from build123d import *

# Parameters (mm, degrees)
SKETCH_1_W               = 40
SKETCH_1_H               = 40
EXTRUDE_1_DEPTH          = 20
SKETCH_2_R               = 3
EXTRUDE_2_DEPTH          = 4.5
SKETCH_4_R               = 2
SKETCH_4_W               = 8
SKETCH_4_H               = 20
EXTRUDE_4_DEPTH          = 2.7
SKETCH_5_W               = 4
SKETCH_5_H               = 7
EXTRUDE_5_DEPTH          = 7
SKETCH_6_W               = 48
SKETCH_6_H               = 20
CUT_EXTRUDE_1_DEPTH      = 27.5
CUT_EXTRUDE_3_DEPTH      = 54.481305145
CUT_EXTRUDE_3_DEPTH_BACK = 54.481305145
SKETCH_7_W               = 40
SKETCH_7_H               = 20
SKETCH_8_W               = 56
SKETCH_8_H               = 5
EXTRUDE_6_DEPTH          = 2.7
SKETCH_9_W               = 56
SKETCH_9_H               = 25
EXTRUDE_7_DEPTH          = 30
CUT_EXTRUDE_4_DEPTH      = 62.878914018
CUT_EXTRUDE_4_DEPTH_BACK = 62.878914018
SKETCH_10_W              = 40
SKETCH_10_H              = 20
CUT_EXTRUDE_5_DEPTH      = 64.232033021
CUT_EXTRUDE_5_DEPTH_BACK = 64.232033021
SKETCH_11_R              = 2
SKETCH_11_R_2            = 2.023853946
CUT_EXTRUDE_6_DEPTH      = 75.500268456
CUT_EXTRUDE_6_DEPTH_BACK = 75.500268456
SKETCH_12_W              = 27.5
SKETCH_12_H              = 18.538560396
SKETCH_13_W              = 56
SKETCH_13_H              = 25
EXTRUDE_8_DEPTH          = 4
SKETCH_14_W              = 36.7
SKETCH_14_H              = 2
EXTRUDE_9_DEPTH          = 56
SKETCH_15_W              = 36.7
SKETCH_15_H              = 2
EXTRUDE_10_DEPTH         = 8
SKETCH_16_W              = 36.7
SKETCH_16_H              = 2
EXTRUDE_11_DEPTH         = 8
CUT_EXTRUDE_7_DEPTH      = 76.918969961
CUT_EXTRUDE_7_DEPTH_BACK = 76.918969961
SKETCH_17_W              = 40.5
SKETCH_17_H              = 30
SKETCH_20_W              = 7.75
SKETCH_20_H              = 22.78217045
CUT_EXTRUDE_9_DEPTH      = 8
SKETCH_21_R              = 1.5
CUT_EXTRUDE_10_DEPTH     = 78.515740337


with BuildPart() as part:
    # Sketch 1 → Extrude 1 (new body)
    with BuildSketch(Plane(origin=(0, 0, 0), x_dir=(1, 0, 0), z_dir=(0, 1, 0))):
        with Locations((20, 20)):
            Rectangle(SKETCH_1_W, SKETCH_1_H)
    extrude(amount=EXTRUDE_1_DEPTH)

    # Sketch 2 → Extrude 2 (add)
    with BuildSketch(Plane.XY):
        with Locations(Location((10, 10, 0), (0, 0, 180))):
            Circle(SKETCH_2_R)
    extrude(amount=EXTRUDE_2_DEPTH)

    # Sketch 4 → Extrude 4 (add)
    # profile 1 of 3: a face of its own
    with BuildSketch(Plane(origin=(0, 0, -12.3), x_dir=(-1, 0, 0), z_dir=(0, 0, -1))):
        with BuildLine():
            Line((-44.5, 17), (-44.5, 20))
            Line((-44.5, 20), (-48, 20))
            Line((-48, 20), (-48, 0))
            Line((-48, 0), (-40, 0))
            Line((-40, 0), (-40, 15))
            Line((-40, 15), (-42.5, 15))
            ThreePointArc((-42.5, 15), (-45.914213562, 13.585786438), (-44.5, 17))
        make_face()
        with Locations((-44.5, 5)):
            Circle(SKETCH_4_R, mode=Mode.SUBTRACT)
    # profile 2 of 3: a face of its own
    with BuildSketch(Plane(origin=(0, 0, -12.3), x_dir=(-1, 0, 0), z_dir=(0, 0, -1))):
        with BuildLine():
            Line((-40, 15), (-40, 20))
            Line((-40, 20), (-44.5, 20))
            Line((-44.5, 20), (-44.5, 17))
            ThreePointArc((-44.5, 17), (-43.085786438, 16.414213562), (-42.5, 15))
            Line((-42.5, 15), (-40, 15))
        make_face()
    # profile 3 of 3: a face of its own
    with BuildSketch(Plane(origin=(0, 0, -12.3), x_dir=(-1, 0, 0), z_dir=(0, 0, -1))):
        with Locations((4, 10)):
            Rectangle(SKETCH_4_W, SKETCH_4_H)
        with Locations((4.5, 5)):
            Circle(SKETCH_4_R, mode=Mode.SUBTRACT)
        with Locations((4.5, 15)):
            Circle(SKETCH_4_R, mode=Mode.SUBTRACT)
    extrude(amount=-EXTRUDE_4_DEPTH)

    # Sketch 5 → Extrude 5 (add)
    with BuildSketch(Plane.ZY):
        with Locations((-35, 10)):
            Rectangle(SKETCH_5_W, SKETCH_5_H)
    extrude(amount=EXTRUDE_5_DEPTH)

    # Sketch 6 → Cut-Extrude 1 (cut)
    with BuildSketch(Plane(origin=(0, 0, -40), x_dir=(-1, 0, 0), z_dir=(0, 0, -1))):
        with Locations((-16, 10)):
            Rectangle(SKETCH_6_W, SKETCH_6_H)
    extrude(amount=-CUT_EXTRUDE_1_DEPTH, mode=Mode.SUBTRACT)

    # Sketch 7 → Cut-Extrude 3 (cut, two sides: drawn at the far end of the back side and taken through both)
    with BuildSketch(Plane.XY.offset(-CUT_EXTRUDE_3_DEPTH_BACK)):
        with Locations((20, 10)):
            Rectangle(SKETCH_7_W, SKETCH_7_H)
    extrude(amount=CUT_EXTRUDE_3_DEPTH + CUT_EXTRUDE_3_DEPTH_BACK, mode=Mode.SUBTRACT)


with BuildPart() as cut_extrude_3_piece_1:
    # of the separate pieces the step leaves, piece 1, a body of its own (cut_extrude_3_pieces)
    add(part.part.solids().sort_by_distance((0, 20, -9.6))[0])



with BuildPart() as cut_extrude_3_piece_2:
    # of the separate pieces the step leaves, piece 2, a body of its own (cut_extrude_3_pieces)
    add(part.part.solids().sort_by_distance((40, 0, -9.6))[0])


with BuildPart() as cut_extrude_3_piece_1_1:
    add(cut_extrude_3_piece_1.part)

    add(cut_extrude_3_piece_2.part)  # Extrude 6 merges Cut-Extrude 3 piece 2
    # Sketch 8 → Extrude 6 (add)
    with BuildSketch(Plane.XY.offset(-9.6)):
        with Locations((20, 22.5)):
            Rectangle(SKETCH_8_W, SKETCH_8_H)
    extrude(amount=-EXTRUDE_6_DEPTH)

    # Sketch 9 → Extrude 7 (add)
    with BuildSketch(Plane(origin=(0, 0, -12.3), x_dir=(-1, 0, 0), z_dir=(0, 0, -1))):
        with Locations((-20, 12.5)):
            Rectangle(SKETCH_9_W, SKETCH_9_H)
    extrude(amount=EXTRUDE_7_DEPTH)

    # Sketch 10 → Cut-Extrude 4 (cut, two sides: drawn at the far end of the back side and taken through both)
    with BuildSketch(Plane.XY.offset(-12.3).offset(-CUT_EXTRUDE_4_DEPTH_BACK)):
        with Locations((20, 10)):
            Rectangle(SKETCH_10_W, SKETCH_10_H)
    extrude(amount=CUT_EXTRUDE_4_DEPTH + CUT_EXTRUDE_4_DEPTH_BACK, mode=Mode.SUBTRACT)

    # Sketch 11 → Cut-Extrude 5 (cut, two sides: drawn at the far end of the back side and taken through both)
    with BuildSketch(Plane.XY.offset(-9.6).offset(-CUT_EXTRUDE_5_DEPTH_BACK)):
        with Locations(Location((-4.5, 15, 0), (0, 0, 180))):
            Circle(SKETCH_11_R)
        with Locations(Location((-4.5, 5, 0), (0, 0, 180))):
            Circle(SKETCH_11_R)
        with Locations((44.5, 15)):
            Circle(SKETCH_11_R_2)
        with Locations(Location((44.5, 5, 0), (0, 0, 180))):
            Circle(SKETCH_11_R)
    extrude(amount=CUT_EXTRUDE_5_DEPTH + CUT_EXTRUDE_5_DEPTH_BACK, mode=Mode.SUBTRACT)

    # Sketch 12 → Cut-Extrude 6 (cut, two sides: drawn at the far end of the back side and taken through both)
    with BuildSketch(Plane(origin=(48, 0, 0), x_dir=(0, 0, -1), z_dir=(1, 0, 0)).offset(-CUT_EXTRUDE_6_DEPTH_BACK)):
        with Locations((27.459022476, 9.269280198)):
            Rectangle(SKETCH_12_W, SKETCH_12_H)
    extrude(amount=CUT_EXTRUDE_6_DEPTH + CUT_EXTRUDE_6_DEPTH_BACK, mode=Mode.SUBTRACT)

    # Sketch 13 → Extrude 8 (add)
    with BuildSketch(Plane(origin=(0, 0, -42.3), x_dir=(-1, 0, 0), z_dir=(0, 0, -1))):
        with Locations((-20, 12.5)):
            Rectangle(SKETCH_13_W, SKETCH_13_H)
    extrude(amount=EXTRUDE_8_DEPTH)

    # Sketch 14 → Extrude 9 (add)
    with BuildSketch(Plane(origin=(48, 0, 0), x_dir=(0, 0, -1), z_dir=(1, 0, 0))):
        with Locations((27.95, -1)):
            Rectangle(SKETCH_14_W, SKETCH_14_H)
    extrude(amount=-EXTRUDE_9_DEPTH)

    # Sketch 15 → Extrude 10 (add)
    with BuildSketch(Plane(origin=(48, 0, 0), x_dir=(0, 0, -1), z_dir=(1, 0, 0))):
        with Locations((27.95, -1)):
            Rectangle(SKETCH_15_W, SKETCH_15_H)
    extrude(amount=EXTRUDE_10_DEPTH)

    # Sketch 16 → Extrude 11 (add)
    with BuildSketch(Plane.ZY.offset(8)):
        with Locations((-27.95, -1)):
            Rectangle(SKETCH_16_W, SKETCH_16_H)
    extrude(amount=EXTRUDE_11_DEPTH)

    # Sketch 17 → Cut-Extrude 7 (cut, two sides: drawn at the far end of the back side and taken through both)
    with BuildSketch(Plane.XZ.offset(-20).offset(-CUT_EXTRUDE_7_DEPTH_BACK)):
        with Locations((20.25, -24.6)):
            Rectangle(SKETCH_17_W, SKETCH_17_H)
    extrude(amount=CUT_EXTRUDE_7_DEPTH + CUT_EXTRUDE_7_DEPTH_BACK, mode=Mode.SUBTRACT)

    # Sketch 20 → Cut-Extrude 9 (cut)
    with BuildSketch(Plane.XZ.offset(2)):
        with Locations((-3.875, -28.208914775)):
            Rectangle(SKETCH_20_W, SKETCH_20_H)
        with Locations((44.375, -28.208914775)):
            Rectangle(SKETCH_20_W, SKETCH_20_H)
    extrude(amount=-CUT_EXTRUDE_9_DEPTH, mode=Mode.SUBTRACT)

    # Sketch 21 → Cut-Extrude 10 (cut, through all)
    with BuildSketch(Plane.XZ.offset(2)):
        with Locations(Location((52.5, -42.3, 0), (0, 0, 270))):
            Circle(SKETCH_21_R)
        with Locations(Location((52.5, -13.6, 0), (0, 0, 270))):
            Circle(SKETCH_21_R)
        with Locations(Location((-12, -13.6, 0), (0, 0, 270))):
            Circle(SKETCH_21_R)
        with Locations(Location((-12, -42.3, 0), (0, 0, 270))):
            Circle(SKETCH_21_R)
    extrude(amount=-CUT_EXTRUDE_10_DEPTH, mode=Mode.SUBTRACT)


solid = cut_extrude_3_piece_1_1.part
Here's how the part is built. I have some questions about the finished solid (model axes, mm). A direction names the side the tool comes from. Coordinates: 2 decimals unless noted, no trailing zeros. Write each loop counter-clockwise with the first axis right and the second up, starting at its lowest first coordinate (ties: lowest second). Pieces come first, ordered by that corner, then holes.
Item 1: Will these pins go through, and if not, where does the flat tip stop? pin 1 (5 mm diameter, centred on x = 10.5, y = 22, fed in from +Z); pin 2 (12 mm diameter, centred on x = 36, z = -23.5, fed in from -Y); pin 3 (8 mm diameter, centred on x = 21, y = 13, fed in from +Z).
Item 2: If we mould it in two halves opening along Y, with no side actions, what happens to faces 6 (the flat face through (18, 0, -40)), 7 (the flat face through (20, 25, -40)), 8 (the flat face through (44, -1, -16.818))? For each: +Y half, -Y half, draft (parallel to the pull), parting line (faces both ways), or undercut.
Item 3: I want a section at D-D on y = 15. Count the separate pieces of the cut face and the enclosed holes in it, and give its area (3 significant figures).
Item 4: I want a section at C-C on y = 10. Write out the boundary of the cut face in (x, z).
Item 5: I want a section at A-A on x = 44.5. Write out the boundary of the cut face in (y, z), and give its area (3 significant figures).
Item 6: I want a section at B-B on z = -35. Write out the boundary of the cut face in (x, y), and give its area (3 significant figures).
Item 7: If I drill on line 1 (Y direction, x = -4.5, z = -41.55); line 2 (X direction, y = 20.25, z = -31.5); line 3 (Y direction, x = -4, z = -41), over which ranges is the centre line in solid material (lowest first)?
Item 8: On a 3-axis mill with a long thin cutter (end or side, diameter ignored), from which of +Z, -Z, +X, -X, +Y, -Y can I reach the whole of each face in a straight line? I mean faces 1 (the flat face through (40.5, 19, -20)), 2 (the cylindrical face through (-2.9, 6.2, -41.8)), 3 (the flat face through (48.25, -1, -28)), 4 (the flat face through (44, 9, -13.709)), 5 (the flat face through (21, 11, -46.3)). Say none if no direction works.
Findings below:
1. pin 1: stops at z = -39.6
1. pin 2: stops at y = 18.54
1. pin 3: stops at z = -42.3
2. face 6: undercut
2. face 7: +Y half
2. face 8: draft
3. separate pieces: 5
3. enclosed holes: 0
3. area: 263 mm2
4. outline: (-8, -46.3) - (48, -46.3) - (48, -41.21) - (40, -41.21) - (40, -42.3) - (0, -42.3) - (0, -41.21) - (-8, -41.21) - close; (-8, -13.71) - (0, -13.71) - (0, -9.6) - (-8, -9.6) - close; (40.5, -13.71) - (48, -13.71) - (48, -9.6) - (40.5, -9.6) - close
5. outline: (-2, -46.3) - (25, -46.3) - (25, -9.6) - (17.02, -9.6) - (17.02, -13.71) - (18.54, -13.71) - (18.54, -41.21) - (17.02, -41.21) - (17.02, -42.3) - (12.98, -42.3) - (12.98, -41.21) - (7, -41.21) - (7, -42.3) - (3, -42.3) - (3, -41.21) - (0, -41.21) - (0, -39.6) - (-2, -39.6) - close; (-2, -16.82) - (0, -16.82) - (0, -13.71) - (3, -13.71) - (3, -9.6) - (-2, -9.6) - close; (7, -13.71) - (12.98, -13.71) - (12.98, -9.6) - (7, -9.6) - close
5. area: 394 mm2
6. outline: (-16, -2) - (-7.75, -2) - (-7.75, 0) - (-16, 0) - close; (-8, 18.54) - (0, 18.54) - (0, 25) - (-8, 25) - close; (40.5, 18.54) - (48, 18.54) - (48, 25) - (40.5, 25) - close; (48.25, -2) - (56, -2) - (56, 0) - (48.25, 0) - close
6. area: 132 mm2
7. line 1: y = -2 to 3, 7 to 13, 17 to 25
7. line 2: x = -8 to 0, 40.5 to 48
7. line 3: y = -2 to 0, 18.54 to 25
8. face 1: +Z, +Y, -Y
8. face 2: +Z
8. face 3: +Y, -Y
8. face 4: +X, -X
8. face 5: -Z, +X, -X, +Y, -Y
